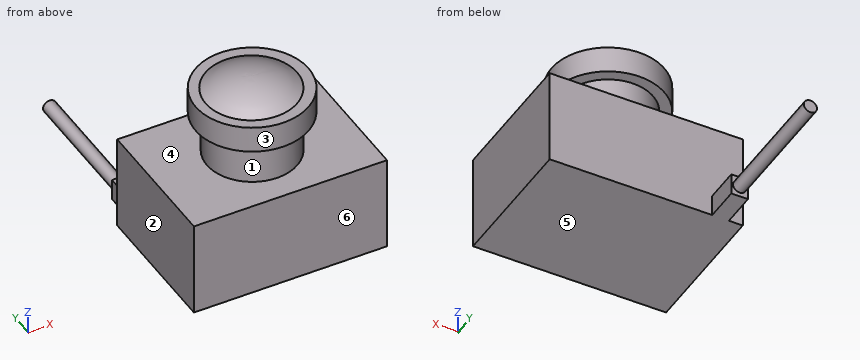
from build123d import *

# Parameters (mm, degrees)
F0_W     = 18
F0_H     = 13
F1_DEPTH = 9
F2_R     = 4.207059
F3_DEPTH = 4
F4_R     = 5.259431
F5_DEPTH = 2.5
F7_DEPTH = 2
F8_R     = 0.61362
F9_DEPTH = 12


with BuildPart() as f1:
    # F0 (on Top) → F1 (new body)
    with BuildSketch(Plane.XY):
        Rectangle(F0_W, F0_H)
    extrude(amount=F1_DEPTH)

    # F2 (on face) → F3 (join)
    with BuildSketch(Plane.XY.offset(9)):
        Circle(F2_R)
    extrude(amount=F3_DEPTH)

    # F4 (on face) → F5 (join)
    with BuildSketch(Plane.XY.offset(13)):
        Circle(F4_R)
    extrude(amount=F5_DEPTH)

    # F6 (on face) → F7 (join)
    with BuildSketch(Plane(origin=(0, 0, 0), x_dir=(1, 0, 0), z_dir=(0, 0, -1))):
        Polygon((-6.154838, -4.973606), (-7.709091, -4.942521), (-7.709091, -9.729618), (-6.154838, -9.729618), align=None)
    extrude(amount=-F7_DEPTH)

    # F8 (on face) → F9 (join)
    with BuildSketch(Plane(origin=(0, 9.729618, 0), x_dir=(-1, 0, 0), z_dir=(0, 1, 0))):
        with Locations((6.931964, 1)):
            Circle(F8_R)
    extrude(amount=F9_DEPTH)

    # F10 (on Front) → F11 (revolve)
    with BuildSketch(Plane.XZ):
        with BuildLine():
            Line((4.402904, 14.748257), (4.402904, 15.349783))
            ThreePointArc((4.402904, 15.349783), (2.276801, 16.411373), (-0.072503, 16.769225))
            Line((-0.072503, 16.769225), (-0.072503, 14.748257))
            Line((-0.072503, 14.748257), (4.402904, 14.748257))
        make_face()
    revolve(axis=Axis((-0.072503, 0, 15.758741), (0, 0, -1)))


solid = f1.part
Model file for the job. Use its own axes, mm. Face numbers are marked on the shaded views. A direction names the side the tool comes from. Give positions to 0.01 mm unless a question says otherwise; leave off trailing zeros. Loops run counter-clockwise (first coordinate to the right, second up) from the corner with the lowest first, then second, coordinate; pieces in that order, holes last.
Item 1: Slice it at C-C (x = 6.5). Write the cut outline in (y, z).
Check values:
outline: (-6.5, 0) - (6.5, 0) - (6.5, 9) - (-6.5, 9) - close
Item 2: Drill centre lines: line 1 along Y through (x, z) = (7, 5); line 2 along X through (y, z) = (7.25, 1.5); line 3 along Z through (x, y) = (3.5, 4.75). Where is each one in solid material? Low to high.
Check values:
line 1: y = -6.5 to 6.5
line 2: x = -7.71 to -6.15
line 3: z = 0 to 9
Item 3: Which spindle directions (+Z, -Z, +X, -X, +Y, -Y) get a long thin tool onto all of the face, cutting with end or side? Do the marked faces 1, 2 and 3. Say none if no direction does.
Check values:
face 1: none
face 2: +Z, -Z, -X, +Y, -Y
face 3: +Z
Item 4: Slice it at A-A (z = 1). Write the cut outline in (x, y), plus the area to 3 significant figures.
Check values:
outline: (-9, -6.5) - (9, -6.5) - (9, 6.5) - (-6.15, 6.5) - (-6.15, 9.73) - (-6.32, 9.73) - (-6.32, 21.73) - (-7.55, 21.73) - (-7.55, 9.73) - (-7.71, 9.73) - (-7.71, 6.5) - (-9, 6.5) - close
area: 254 mm2
Item 5: Slice it at B-B (y = 8.5). Write the cut outline in (x, z), plus the area to 3 significant figures.
Check values:
outline: (-7.71, 0) - (-6.15, 0) - (-6.15, 2) - (-7.71, 2) - close
area: 3.11 mm2
Item 6: Slice it at D-D (z = 11.5). Write the cut outline in (x, y).
Check values:
outline: circle Ø8.41 at (0, 0)
Item 7: Drop flat-ended pins along their axis: P1, Ø1.6, axis at y = 8, z = 0.5, coming from the +X side; P2, Ø1.2, axis at x = -7, y = 8.5, coming from the +Z side; P3, Ø4.5, axis at x = 0, z = 3, coming from the +Y side. Give the stop position or say it passes through.
Check values:
P1: stops at x = -6.15
P2: stops at z = 2
P3: stops at y = 6.5
Item 8: Mould opens along Z. For the marked faces 4, 5 and 6 say: +Z half, -Z half, draft (parallel to the pull), parting line (faces both ways), or undercut.
Check values:
face 4: undercut
face 5: -Z half
face 6: draft
